from build123d import *

# Parameters (mm, degrees)
F0_R        = 4.35
F1_DEPTH    = 20
F2_R        = 3.25
F3_DEPTH    = 25
F1_FACE_R   = 4.35
F1_FACE_R_2 = 3.25


with BuildPart() as f1:
    # F0 (on Top) → F1 (new body)
    with BuildSketch(Plane.XY):
        Circle(F0_R)
    extrude(amount=F1_DEPTH)

    # F2 (on face) → F3 (cut)
    with BuildSketch(Plane.XY.offset(20)):
        Circle(F2_R)
    extrude(amount=-F3_DEPTH, mode=Mode.SUBTRACT)

    # F5: sweep along a path in F4
    with BuildLine(Plane.XZ) as f5_path:
        ThreePointArc((0, 20), (-60, 80), (-120, 20))
    # F1_face (on face) → F5 (sweep)
    with BuildSketch(Plane.XY.offset(20)):
        Circle(F1_FACE_R)
        Circle(F1_FACE_R_2, mode=Mode.SUBTRACT)
    sweep(path=f5_path.line)


solid = f1.part
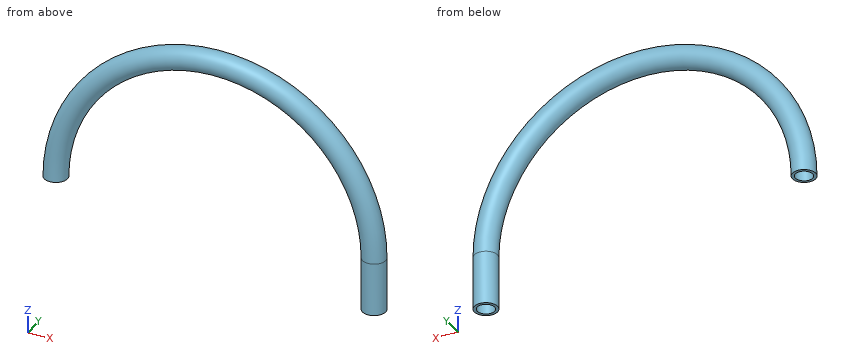
Read the model definition and answer for the solid it produces. Units are mm, in the model's axes. Round coordinates to 2 decimals unless told otherwise and drop trailing zeros. Loops run counter-clockwise (first coordinate to the right, second up) from the corner with the lowest first, then second, coordinate; pieces in that order, holes last. Notation, with made-up numbers: (-30, 73) - (0, 73) arc R12 cw to (0, 85) - close; hole circle Ø5 at (71, 49). An arc over 180 degrees is marked (long way). One line per question, with ' | ' between items. Start each with the question number.
Q1. Section B-B on z = 16.5 is taken. Give the vertices of the cut face in (x, y).
Q2. Section C-C on z = 63 is taken. Count the separate pieces of the cut face and the enclosed holes in it, plus the area to 3 significant figures.
Q3. Flat-ended cylindrical pins translate along their axes: pin 1 (5 mm diameter, centred on x = 0, y = 0, fed in from +Z); pin 2 (1.5 mm diameter, centred on x = -25.5, y = 0, fed in from +Z); pin 3 (5 mm diameter, centred on y = 3.5, z = 71, fed in from +X). Find the tip coordinate at first contact, or state that the pin passes through.
Q4. Find the intervals of material crossed by L1, parallel to Y at x = 0, z = 6; L2, parallel to X at y = -2, z = 62.5; L3, parallel to X at y = -0.25, z = 71, in increasing order.
Q5. Section A-A on y = 0 is taken. Give the vertices of the cut face in (x, z).
Established:
1) outline: circle Ø8.7 at (0, 0); hole circle Ø6.5 at (0, 0)
2) separate pieces: 2 | enclosed holes: 2 | area: 75.8 mm²
3) pin 1: z = 48.89 | pin 2: z = 74.79 | pin 3: x = -19.04
4) L1: -4.35 to -3.25, 3.25 to 4.35 | L2: -107.67 to -105.91, -98.64 to -96.68, -23.32 to -21.36, -14.09 to -12.33 | L3: -99.23 to -97.39, -84.91 to -82.29, -37.71 to -35.09, -22.61 to -20.77
5) outline: (-124.35, 20) - (-123.25, 20) arc R63.25 cw to (3.25, 20) - (3.25, 0) - (4.35, 0) - (4.35, 20) arc R64.35 ccw to start; (-116.75, 20) - (-115.65, 20) arc R55.65 cw to (-4.35, 20) - (-4.35, 0) - (-3.25, 0) - (-3.25, 20) arc R56.75 ccw to start
